Here's how the part is built. I have some questions about the finished solid (model axes, mm). Face numbers are marked on the shaded views. A direction names the side the tool comes from. Round coordinates to 2 decimals unless told otherwise and drop trailing zeros. Order: outer loops, then holes, each group sorted by start corner. A loop starts at its lowest first (then second) coordinate and runs counter-clockwise, first axis right, second up. Notation, with made-up numbers: M -36,81.25 L -7,81.25 A23 cw -7,106.25 Z; hole C 43.5,88.5 d1. An arc over 180 degrees is marked long. Write each question's results on one line, items separated by ' | '. Start each with the question number.
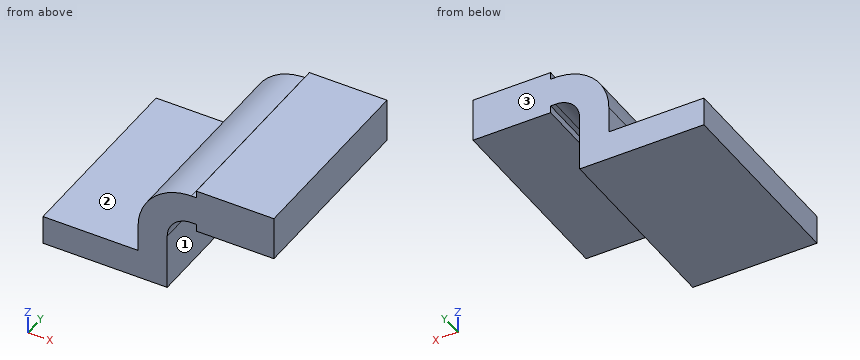
```python
from build123d import *

# Parameters (mm, degrees)
F0_W     = 24.6055256037
F0_H     = 4.7752
F0_H_2   = 4.7498
F0_H_3   = 19.05
F1_DEPTH = 63.5


with BuildPart() as f1:
    # F0 (on Front) → F1 (new body, symmetric)
    with BuildSketch(Plane.XZ):
        with BuildLine():
            ThreePointArc((56.515, 61.9252), (55.3078445888, 61.9043315723), (54.1021317795, 61.8417512277))
            add(Edge.make_bspline(
                [(54.1021317795, 61.8417512277), (54.9069035944, 61.8717262764), (55.7112681225, 61.8994528512), (56.515, 61.9252)],
                knots=[108.1784271966, 108.1784271966, 108.1784271966, 108.1784271966, 110.3851212122, 110.3851212122, 110.3851212122, 110.3851212122], degree=3))
        make_face()
        Polygon((-40.64, -9.525), (40.64, -9.525), (40.64, 9.525), (21.59, 9.525), (-40.64, 9.525), align=None)
        with Locations((71.9927628018, 40.4876)):
            Rectangle(F0_W, F0_H)
        with Locations((71.9927628018, 64.3001)):
            Rectangle(F0_W, F0_H_2)
        Polygon((84.2955256037, 61.9252), (84.2955256037, 42.8752), (84.2955256037, 38.1), (110.49, 38.1), (110.49, 66.675), (84.2955256037, 66.675), align=None)
        with Locations((71.9927628018, 52.4002)):
            Rectangle(F0_W, F0_H_3)
        with BuildLine():
            Line((21.59, 9.525), (40.64, 9.525))
            Line((40.64, 9.525), (40.64, 27.0002))
            ThreePointArc((40.64, 27.0002), (45.2896798487, 38.2255201513), (56.515, 42.8752))
            Line((56.515, 42.8752), (59.69, 42.8752))
            Line((59.69, 42.8752), (59.69, 61.9252))
            Line((59.69, 61.9252), (56.515, 61.9252))
            add(Edge.make_bspline(
                [(54.1021317795, 61.8417512277), (54.9069035944, 61.8717262764), (55.7112681225, 61.8994528512), (56.515, 61.9252)],
                knots=[108.1784271966, 108.1784271966, 108.1784271966, 108.1784271966, 110.3851212122, 110.3851212122, 110.3851212122, 110.3851212122], degree=3))
            ThreePointArc((54.1021317795, 61.8417512277), (30.9804640966, 50.827560349), (21.59, 27.0002))
            Line((21.59, 27.0002), (21.59, 9.525))
        make_face()
    extrude(amount=F1_DEPTH, both=True)


solid = f1.part
```
(1) I want a section at C-C on x = 89. Write out the boundary of the cut face in (y, z) (3 decimals).
(2) I'm going to push flat-ended pins straight in: pin 1 Ø18.5 at (y, z) = (-14, 16) entering from +X; pin 2 Ø1.4 at (y, z) = (14, 40.5) entering from -X; pin 3 Ø1.6 at (x, y) = (58.5, 22.5) entering from +Z. Where does each tip first touch, or does it pass through?
(3) On a 3-axis mill with a long thin cutter (end or side, diameter ignored), from which of +Z, -Z, +X, -X, +Y, -Y can I reach the whole of each face in a straight line? I mean the marked faces 1, 2 and 3. Say none if no direction works.
(4) I want a section at B-B on z = -0.5. Write out the boundary of the cut face in (x, y), and give its area (3 significant figures).
(5) I want a section at A-A on y = 46.5. Write out the boundary of the cut face in (x, z) (3 decimals).
(6) Please list where these lines run through material, in increasing order: line 1 (Z direction, x = -11, y = -21.5) (3 decimals); line 2 (X direction, y = -29, z = 63); line 3 (X direction, y = -10, z = 5).
Solutions:
1) outline: M -63.5,38.1 L 63.5,38.1 L 63.5,66.675 L -63.5,66.675 Z
2) pin 1: x = 40.64 | pin 2: x = 24.02 | pin 3: z = 61.93
3) face 1: -Z, +X, +Y, -Y | face 2: +Z, -X, +Y, -Y | face 3: +Z, -Z, +X, -X, +Y
4) outline: M -40.64,-63.5 L 40.64,-63.5 L 40.64,63.5 L -40.64,63.5 Z | area: 10,300 mm^2
5) outline: M -40.64,-9.525 L 40.64,-9.525 L 40.64,27 A15.875 cw 56.515,42.875 L 59.69,42.875 L 59.69,38.1 L 110.49,38.1 L 110.49,66.675 L 59.69,66.675 L 59.69,61.925 L 56.515,61.925 A34.925 ccw 21.59,27 L 21.59,9.525 L -40.64,9.525 Z
6) line 1: -9.525 to 9.525 | line 2: 59.69 to 110.49 | line 3: -40.64 to 40.64
